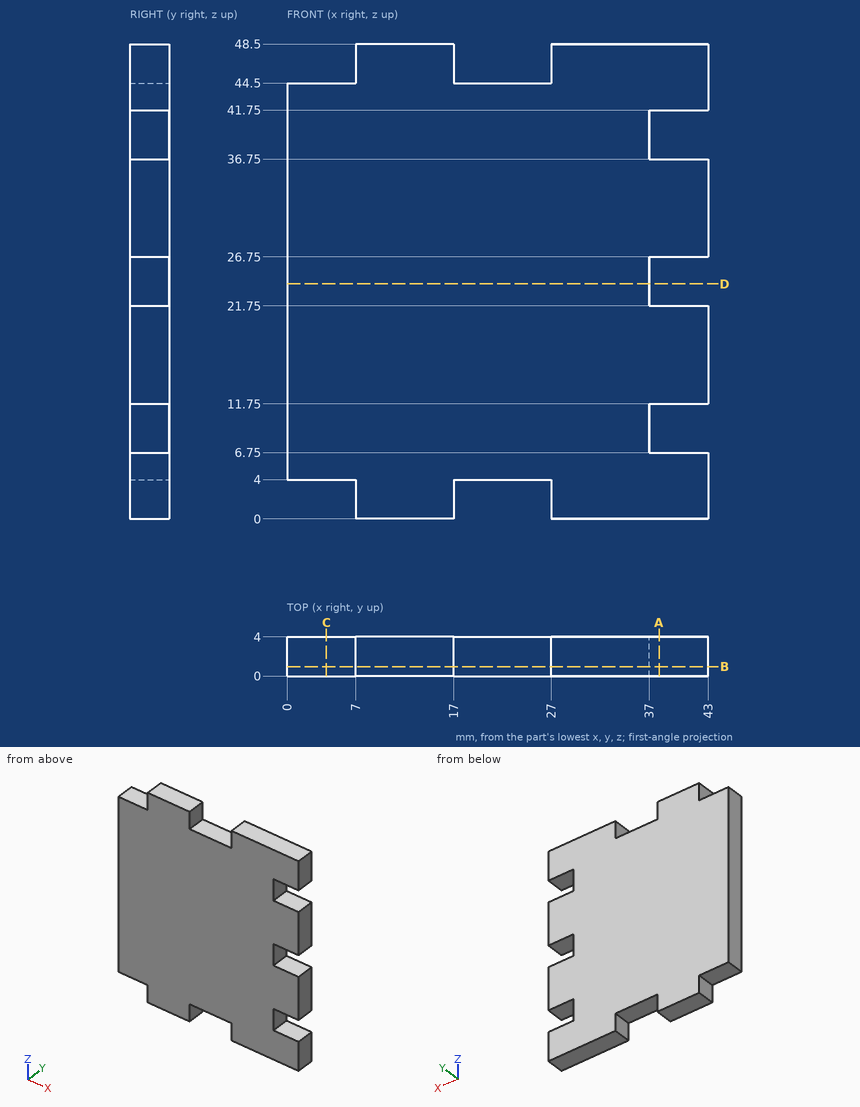
Design review of the part shown in the three views and the two pictorial views. Dimensions are in mm from the part's minimum x, y and z. Round coordinates to 2 decimals unless told otherwise and drop trailing zeros. Write each loop counter-clockwise with the first axis right and the second up, starting at its lowest first coordinate (ties: lowest second). Pieces come first, ordered by that corner, then holes. Notation, with made-up numbers: (86, -32) -> (97, -32) arc R32 cw to (97, 2) -> close; hole circle Ø1 at (51, -24.5). An arc over 180 degrees is marked (long way). One line per question, with ' | ' between items. Start each with the question number.
1) Add section B-B (y = 0.95). Write out the cut boundary in (x, z), and give its area (3 significant figures).
2) Add section D-D (z = 24). Write out the cut boundary in (x, y).
3) Add section A-A (x = 38). Write out the cut boundary in (y, z), and give its area (3 significant figures).
4) Add section C-C (x = 4). Write out the cut boundary in (y, z), and give its area (3 significant figures).
5) Wall thickness on line 1 along X through (y, z) = (0.45, 46.5); line 2 along X through (y, z) = (1.65, 7); line 3 along Z through (x, y) = (19.5, 2.95): over which ranges is each line inside the solid? List them lowest first.
6) For pin 1 Ø2 at (x, y) = (22, 2) entering from +Z; pin 2 Ø1.2 at (y, z) = (1.5, 46.5) entering from -X; pin 3 Ø2 at (y, z) = (2.5, 25) entering from +X; pin 4 Ø1.2 at (x, y) = (39, 3) entering from -Z, all flat-tipped, find the tip position at first contact; note any pin that passes through.
Reported:
1) outline: (0, 4) -> (7, 4) -> (7, 0) -> (17, 0) -> (17, 4) -> (27, 4) -> (27, 0) -> (43, 0) -> (43, 6.75) -> (37, 6.75) -> (37, 11.75) -> (43, 11.75) -> (43, 21.75) -> (37, 21.75) -> (37, 26.75) -> (43, 26.75) -> (43, 36.75) -> (37, 36.75) -> (37, 41.75) -> (43, 41.75) -> (43, 48.5) -> (27, 48.5) -> (27, 44.5) -> (17, 44.5) -> (17, 48.5) -> (7, 48.5) -> (7, 44.5) -> (0, 44.5) -> close | area: 1,860 mm²
2) outline: (0, 0) -> (37, 0) -> (37, 4) -> (0, 4) -> close
3) outline: (0, 0) -> (4, 0) -> (4, 6.75) -> (0, 6.75) -> close; (0, 11.75) -> (4, 11.75) -> (4, 21.75) -> (0, 21.75) -> close; (0, 26.75) -> (4, 26.75) -> (4, 36.75) -> (0, 36.75) -> close; (0, 41.75) -> (4, 41.75) -> (4, 48.5) -> (0, 48.5) -> close | area: 134 mm²
4) outline: (0, 4) -> (4, 4) -> (4, 44.5) -> (0, 44.5) -> close | area: 162 mm²
5) line 1: x = 7 to 17, 27 to 43 | line 2: x = 0 to 37 | line 3: z = 4 to 44.5
6) pin 1: stops at z = 44.5 | pin 2: stops at x = 7 | pin 3: stops at x = 37 | pin 4: stops at z = 0
